from build123d import *

# Parameters (mm, degrees)
BOSS_EXTRU_1_DEPTH      = 40
ENL_V_MAT_EXTRU_1_REACH = 42
ESQUISSE3_R             = 3
ENL_V_MAT_EXTRU_2_REACH = 42
ESQUISSE4_R             = 3
ENL_V_MAT_EXTRU_4_REACH = 37.2
ESQUISSE9_W             = 10
ESQUISSE9_H             = 10
ENL_V_MAT_EXTRU_5_REACH = 37.2
ESQUISSE10_W            = 10
ESQUISSE10_H            = 10


with BuildPart() as part:
    # Esquisse2 → Boss.-Extru.1 (new body)
    with BuildSketch(Plane.XY):
        Polygon((0, 0), (0, 40), (40, 0), align=None)
    extrude(amount=BOSS_EXTRU_1_DEPTH)

    # Esquisse3 → Enlèv. mat.-Extru.1 (cut, up to next)
    with BuildSketch(Plane.XZ, mode=Mode.PRIVATE) as enl_v_mat_extru_1_sk1:
        with Locations((30, 20)):
            Circle(ESQUISSE3_R)
    enl_v_mat_extru_1_tool1 = extrude(enl_v_mat_extru_1_sk1.sketch, amount=-ENL_V_MAT_EXTRU_1_REACH, mode=Mode.PRIVATE) & part.part
    add(enl_v_mat_extru_1_tool1.solids().sort_by_distance((30, 0, 20))[0], mode=Mode.SUBTRACT)

    # Esquisse4 → Enlèv. mat.-Extru.2 (cut, up to next)
    with BuildSketch(Plane.ZY, mode=Mode.PRIVATE) as enl_v_mat_extru_2_sk1:
        with Locations((20, 30)):
            Circle(ESQUISSE4_R)
    enl_v_mat_extru_2_tool1 = extrude(enl_v_mat_extru_2_sk1.sketch, amount=-ENL_V_MAT_EXTRU_2_REACH, mode=Mode.PRIVATE) & part.part
    add(enl_v_mat_extru_2_tool1.solids().sort_by_distance((0, 30, 20))[0], mode=Mode.SUBTRACT)

    # Esquisse9 → Enlèv. mat.-Extru.4 (cut, up to next)
    with BuildSketch(Plane.ZY.offset(-4.8), mode=Mode.PRIVATE) as enl_v_mat_extru_4_sk1:
        with Locations((20, 30)):
            Rectangle(ESQUISSE9_W, ESQUISSE9_H)
    enl_v_mat_extru_4_tool1 = extrude(enl_v_mat_extru_4_sk1.sketch, amount=-ENL_V_MAT_EXTRU_4_REACH, mode=Mode.PRIVATE) & part.part
    add(enl_v_mat_extru_4_tool1.solids().sort_by_distance((4.8, 30, 20))[0], mode=Mode.SUBTRACT)

    # Esquisse10 → Enlèv. mat.-Extru.5 (cut, up to next)
    with BuildSketch(Plane(origin=(0, 4.8, 0), x_dir=(0, 0, 1), z_dir=(0, -1, 0)), mode=Mode.PRIVATE) as enl_v_mat_extru_5_sk1:
        with Locations((20, -30)):
            Rectangle(ESQUISSE10_W, ESQUISSE10_H)
    enl_v_mat_extru_5_tool1 = extrude(enl_v_mat_extru_5_sk1.sketch, amount=-ENL_V_MAT_EXTRU_5_REACH, mode=Mode.PRIVATE) & part.part
    add(enl_v_mat_extru_5_tool1.solids().sort_by_distance((30, 4.8, 20))[0], mode=Mode.SUBTRACT)


solid = part.part
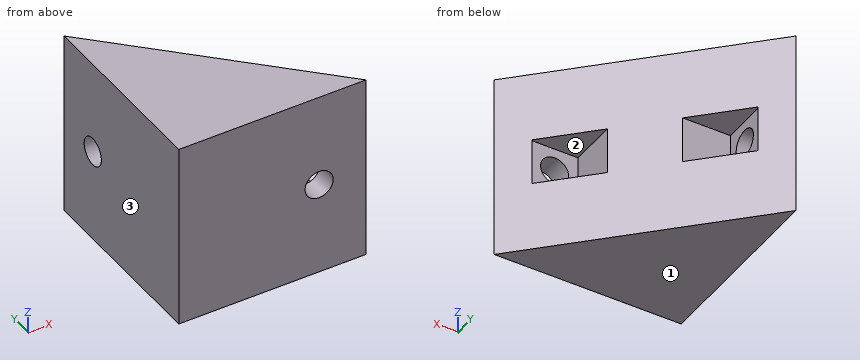
Model file for the job. Use its own axes, mm. Face numbers are marked on the shaded views. Give positions to 0.01 mm unless a question says otherwise; leave off trailing zeros. Write each loop counter-clockwise with the first axis right and the second up, starting at its lowest first coordinate (ties: lowest second). Pieces come first, ordered by that corner, then holes. Notation, with made-up numbers: (49.5, 55.5) -> (94.5, 55.5) arc R17 ccw to (94.5, 81.5) -> close; hole circle Ø2 at (2, 57.25). An arc over 180 degrees is marked (long way). Write item = value, one per line.
(1) Slice it at C-C, the plane z = 20. Give the cut face in (x, y).
Determined:
outline = (0, 0) -> (27, 0) -> (27, 4.8) -> (25, 4.8) -> (25, 15) -> (15, 25) -> (4.8, 25) -> (4.8, 27) -> (0, 27) -> close; (0, 33) -> (4.8, 33) -> (4.8, 35) -> (5, 35) -> (0, 40) -> close; (33, 0) -> (40, 0) -> (35, 5) -> (35, 4.8) -> (33, 4.8) -> close
(2) Slice it at D-D, the plane z = 24. Give the cut face in (x, y).
Determined:
outline = (0, 0) -> (40, 0) -> (35, 5) -> (35, 4.8) -> (25, 4.8) -> (25, 15) -> (15, 25) -> (4.8, 25) -> (4.8, 35) -> (5, 35) -> (0, 40) -> close
(3) Mould opens along Z. For the marked faces 1, 2 and 3 say: released by +Z, released by -Z, zero draft, split by the parting line, or undercut.
Determined:
face_1 = released by -Z
face_2 = undercut
face_3 = zero draft
(4) Probe line 1 along Z through (x, y) = (30, 3.6); line 2 along Y through (x, z) = (15, 25); line 3 along Y through (x, z) = (1.3, 20). List the from-to ranges inside material, lowest first.
Determined:
line_1 = 0 to 17, 23 to 40
line_2 = 0 to 25
line_3 = 0 to 27, 33 to 38.7
(5) Slice it at A-A, the plane y = 30. Give the cut face in (x, z).
Determined:
outline = (0, 0) -> (10, 0) -> (10, 15) -> (4.8, 15) -> (4.8, 17) -> (0, 17) -> close; (0, 23) -> (4.8, 23) -> (4.8, 25) -> (10, 25) -> (10, 40) -> (0, 40) -> close
(6) Flat gauge pins, fed straight in: P1, Ø6, axis at x = 17.5, z = 9, coming from the -Y side; P2, Ø3, axis at y = 6.5, z = 29, coming from the +X side; P3, Ø3, axis at x = 8.5, z = 21, coming from the +Y side; P4, Ø6, axis at y = 15.5, z = 16.5, coming from the +X side. Where does each tip first touch, or does it go through?
Determined:
P1 = 0
P2 = 35
P3 = 25
P4 = 27.1
